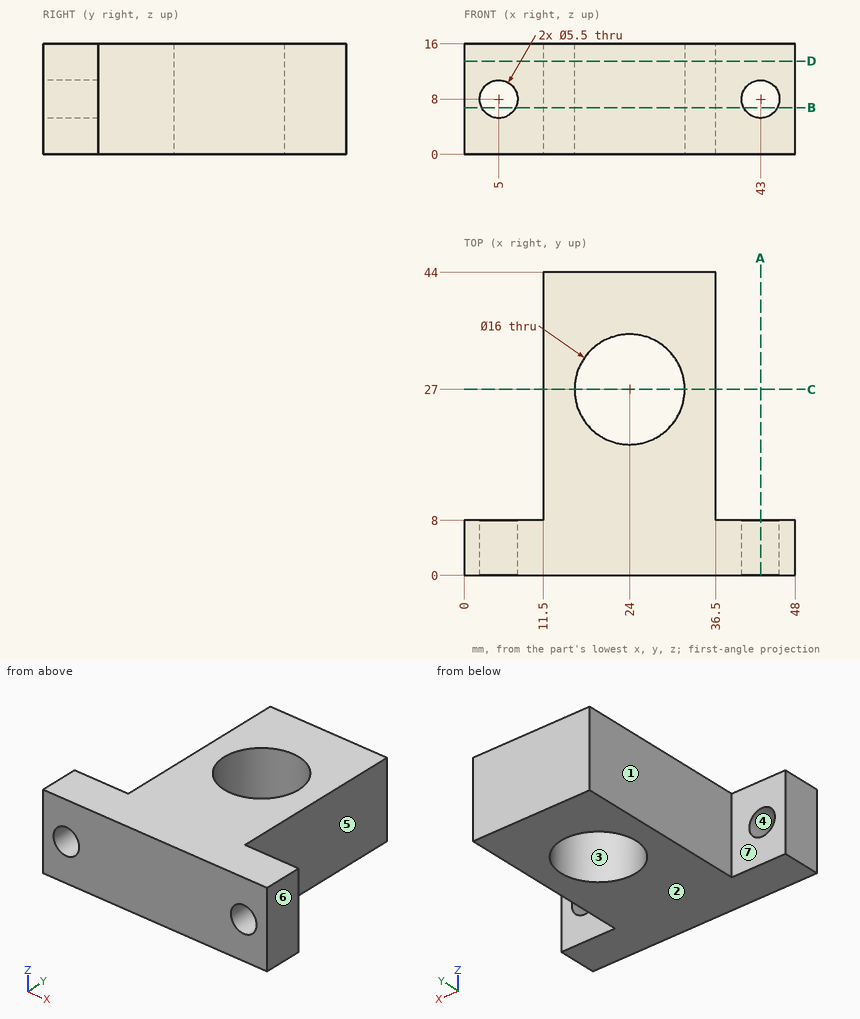
Geometry check sheet. Reference: drawing and pictorial views, mm from the part's lowest x, y, z. A direction names the side the tool comes from. Coordinates: 2 decimals unless noted, no trailing zeros. Order: outer loops, then holes, each group sorted by start corner. A loop starts at its lowest first (then second) coordinate and runs counter-clockwise, first axis right, second up.
Item 1: Scan lines: line 1 along X through (y, z) = (2.75, 8); line 2 along Y through (x, z) = (24, 8.25); line 3 along X through (y, z) = (17, 13.5). Record each from-to range of solid material in increasing order.
Item 2: Section check A-A (x = 43). Enter the section's corners in (y, z), plus the area to 3 significant figures.
Item 3: Section check B-B (z = 6.75). Enter the section's corners in (x, y), plus the area to 3 significant figures.
Item 4: Section check C-C (y = 27). Enter the section's corners in (x, z).
Item 5: Mould release check, pull along X, two halves, no side actions. Record for the marked faces 1, 2, 3 and 4: released by +X, released by -X, zero draft, split by the parting line, or undercut.
Item 6: Depth check by flat-ended pin: pin 1 (2 mm diameter, centred on x = 9.5, y = 37, fed in from -Z); pin 2 (3.5 mm diameter, centred on x = 7.5, z = 5.5, fed in from +Y); pin 3 (5 mm diameter, centred on y = 27.5, z = 7, fed in from +X). Enter the tip coordinate at first touch or a pass-through.
Item 7: Section check D-D (z = 13.5). Enter the section's corners in (x, y), plus the area to 3 significant figures.
Item 8: Tool access check on the marked faces 5, 6 and 7. Record the directions out of +Z, -Z, +X, -X, +Y, -Y that give a thin tool (end or side, any length) a straight path to the whole face; none if there is none.
Check sheet entries:
1. line 1: x = 0 to 2.25, 7.75 to 40.25, 45.75 to 48
1. line 2: y = 0 to 19, 35 to 44
1. line 3: x = 11.5 to 36.5
2. outline: (0, 0) - (8, 0) - (8, 5.25) - (0, 5.25) - close; (0, 10.75) - (8, 10.75) - (8, 16) - (0, 16) - close
2. area: 84.0 mm2
3. outline: (0, 0) - (2.55, 0) - (2.55, 8) - (0, 8) - close; (7.45, 0) - (40.55, 0) - (40.55, 8) - (36.5, 8) - (36.5, 44) - (11.5, 44) - (11.5, 8) - (7.45, 8) - close; (45.45, 0) - (48, 0) - (48, 8) - (45.45, 8) - close; hole circle Ø16 at (24, 27)
3. area: 1,000 mm2
4. outline: (11.5, 0) - (16, 0) - (16, 16) - (11.5, 16) - close; (32, 0) - (36.5, 0) - (36.5, 16) - (32, 16) - close
5. face 1: released by -X
5. face 2: zero draft
5. face 3: undercut
5. face 4: undercut
6. pin 1: passes through
6. pin 2: stops at y = 8
6. pin 3: stops at x = 36.5
7. outline: (0, 0) - (48, 0) - (48, 8) - (36.5, 8) - (36.5, 44) - (11.5, 44) - (11.5, 8) - (0, 8) - close; hole circle Ø16 at (24, 27)
7. area: 1,080 mm2
8. face 5: +Z, -Z, +X, +Y
8. face 6: +Z, -Z, +X, +Y, -Y
8. face 7: +Z, -Z, -X, +Y
